```python
from build123d import *

# Parameters (mm, degrees)
SKETCH_1_W      = 18.2
SKETCH_1_H      = 10.2
EXTRUDE_1_DEPTH = 14.85
SKETCH_3_R      = 0.3
EXTRUDE_2_DEPTH = 3


with BuildPart() as part:
    # Эскиз1 → Бобышка-Вытянуть1 (new body)
    with BuildSketch(Plane(origin=(0, 0, 0), x_dir=(1, 0, 0), z_dir=(0, 1, 0))):
        Rectangle(SKETCH_1_W, SKETCH_1_H)
    extrude(amount=EXTRUDE_1_DEPTH)

    # Эскиз3 → Бобышка-Вытянуть2 (add)
    with BuildSketch(Plane.XZ):
        with Locations(Location((-7.6, 3.8, 0), (0, 0, 90))):
            Circle(SKETCH_3_R)
        with Locations(Location((-7.6, -3.8, 0), (0, 0, 90))):
            Circle(SKETCH_3_R)
        with Locations(Location((6.35, 3.8, 0), (0, 0, 90))):
            Circle(SKETCH_3_R)
        with Locations(Location((4.95, -3.8, 0), (0, 0, 90))):
            Circle(SKETCH_3_R)
        with Locations(Location((7.75, -3.8, 0), (0, 0, 90))):
            Circle(SKETCH_3_R)
    extrude(amount=EXTRUDE_2_DEPTH)


solid = part.part
```
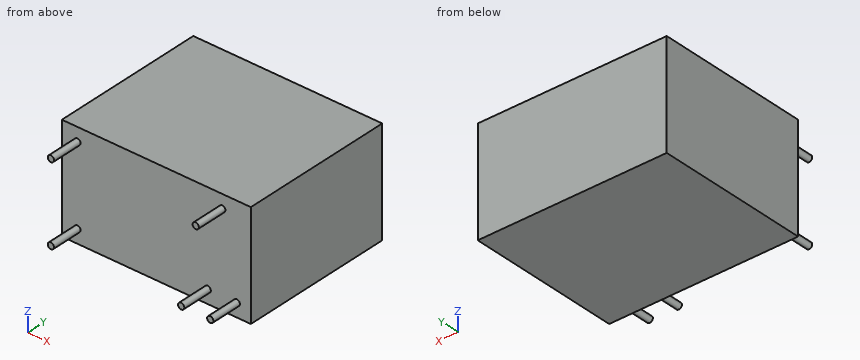
CAD build for the part. Positions are in the model's coordinates, mm. Give positions to 0.01 mm unless a question says otherwise; leave off trailing zeros. Order: outer loops, then holes, each group sorted by start corner. A loop starts at its lowest first (then second) coordinate and runs counter-clockwise, first axis right, second up.
(1) Drill centre line: L1, parallel to Y at x = 8, z = -1. Where is it in solid material? Low to high.
(2) Saw through at C-C, the plane z = -0.75. Give the cut face in (x, y), then the cut area to 3 significant figures.
(3) Saw through at D-D, the plane x = -2.5. Give the cut face in (y, z).
(4) Saw through at A-A, the plane y = -0.5. Give the cut face in (x, z).
(5) Saw through at B-B, the plane x = 6.35. Give the cut face in (y, z).
(6) Flat gauge pin, fed straight in: pin 1 (5 mm diameter, centred on x = -1.5, z = -1, fed in from -Y). Where does the tip first touch, or does it go through?
Results found:
1. L1: y = 0 to 14.85
2. outline: (-9.1, 0) - (9.1, 0) - (9.1, 14.85) - (-9.1, 14.85) - close
2. area: 270 mm2
3. outline: (0, -5.1) - (14.85, -5.1) - (14.85, 5.1) - (0, 5.1) - close
4. outline: circle Ø0.6 at (-7.6, -3.8); circle Ø0.6 at (-7.6, 3.8); circle Ø0.6 at (4.95, -3.8); circle Ø0.6 at (6.35, 3.8); circle Ø0.6 at (7.75, -3.8)
5. outline: (-3, 3.5) - (0, 3.5) - (0, -5.1) - (14.85, -5.1) - (14.85, 5.1) - (0, 5.1) - (0, 4.1) - (-3, 4.1) - close
6. pin 1: stops at y = 0
